Answer from the drawing. Dimensions are ordinates in mm from the lowest x, y and z of the part. Give positions to 0.01 mm unless a question says otherwise; leave off trailing zeros. Order: outer loops, then holes, each group sorted by start corner. A loop starts at its lowest first (then second) coordinate and runs counter-clockwise, first axis right, second up.
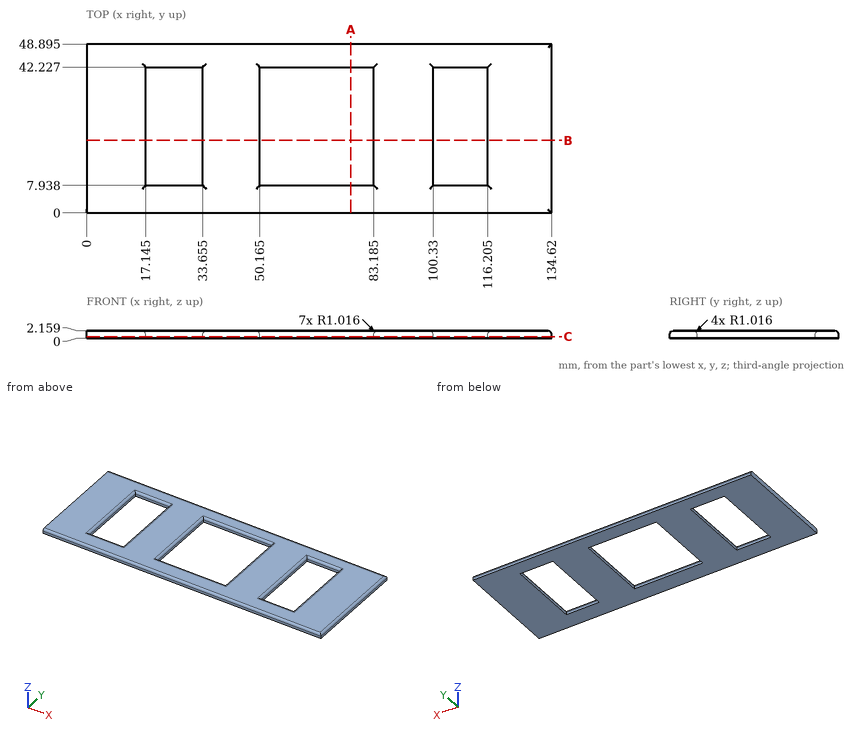
1) Given pin 1 (1.5 mm diameter, centred on x = 111, y = 8, fed in from +Z) (1 decimal); pin 2 (1 mm diameter, centred on x = 18, y = 40, fed in from -Z), each flat-ended and moving along its own axis, determine where each tip first touches the part or whether it passes through.
Final values:
pin 1: stops at z = 2.1
pin 2: passes through
2) The part is cut by section C-C on z = 0.5. Determine the outline of the cut face in (x, y) (1 decimal), and give its area (3 significant figures).
Final values:
outline: (0, 0) - (134.6, 0) - (134.6, 48.9) - (0, 48.9) - close; hole (17.1, 7.9) - (33.7, 7.9) - (33.7, 42.2) - (17.1, 42.2) - close; hole (50.2, 7.9) - (83.2, 7.9) - (83.2, 42.2) - (50.2, 42.2) - close; hole (100.3, 7.9) - (116.2, 7.9) - (116.2, 42.2) - (100.3, 42.2) - close
area: 4,340 mm2
3) The part is cut by section B-B on y = 21. Count the separate pieces of the cut face and the enclosed holes in it, and give its area (3 significant figures).
Final values:
separate pieces: 4
enclosed holes: 0
area: 148 mm2
4) Consider L1, parallel to X at y = 31, z = 1.05 (1 decimal); L2, parallel to X at y = 8.5, z = 2.05 (1 decimal); L3, parallel to Y at x = 74.5, z = 0.3 (1 decimal). Determine where each line is inside the solid, lowest interval first.
Final values:
L1: x = 0 to 17.1, 33.7 to 50.2, 83.2 to 100.3, 116.2 to 134.6
L2: x = 0 to 16.6, 34.2 to 49.6, 83.7 to 99.8, 116.8 to 134.1
L3: y = 0 to 7.9, 42.2 to 48.9
5) The part is cut by section A-A on x = 76.5. Determine the outline of the cut face in (y, z) (1 decimal).
Final values:
outline: (0, 0) - (7.9, 0) - (7.9, 1.1) arc R1 ccw to (6.9, 2.2) - (1, 2.2) arc R1 ccw to (0, 1.1) - close; (42.2, 0) - (48.9, 0) - (48.9, 1.1) arc R1 ccw to (47.9, 2.2) - (43.2, 2.2) arc R1 ccw to (42.2, 1.1) - close
